Here's how the part is built. I have some questions about the finished solid (model axes, mm). Face numbers are marked on the shaded views. A direction names the side the tool comes from. Give positions to 0.01 mm unless a question says otherwise; leave off trailing zeros. Write each loop counter-clockwise with the first axis right and the second up, starting at its lowest first coordinate (ties: lowest second). Pieces come first, ordered by that corner, then holes. Notation, with made-up numbers: (9.5, -33.75) - (26.5, -33.75) arc R30 cw to (26.5, -10.75) - close; hole circle Ø3 at (-5.75, 29). An arc over 180 degrees is marked (long way). One line per item, written item: value. Start each with the question number.
1) I'm going to push flat-ended pins straight in: P1, Ø2.5, axis at x = 7, z = -3, coming from the +Y side; P2, Ø1.5, axis at y = 1, z = 6.5, coming from the -X side; P3, Ø1, axis at y = 0, z = 5, coming from the -X side. Where does each tip first touch, or does it pass through?
2) Imagine slicing it at B-B on z = 7. Write out the boundary of the cut face in (x, y).
3) Imagine slicing it at A-A on y = -0.8. Count the separate pieces of the cut face and the enclosed holes in it, plus the area to 3 significant figures.
4) On a 3-axis mill with a long thin cutter (end or side, diameter ignored), from which of +Z, -Z, +X, -X, +Y, -Y can I reach the whole of each face in a straight line? I mean the marked faces 1 and 2. Say none if no direction works.
5) Imagine slicing it at D-D on x = 4. Write out the boundary of the cut face in (y, z).
6) Please list where these lines run through material, in increasing order: L1, parallel to X at y = -0.2, z = 0; L2, parallel to X at y = 0.4, z = -3; L3, parallel to X at y = -0.1, z = 7. Write a range as [from, to].
7) Imagine slicing it at C-C on x = 7. Write out the boundary of the cut face in (y, z), plus the area to 3 significant figures.
8) We'd pull the mould along X, two halves only. Please class the marked faces 3, 4 and 5: +X half, -X half, draft (parallel to the pull), parting line (faces both ways), or undercut.
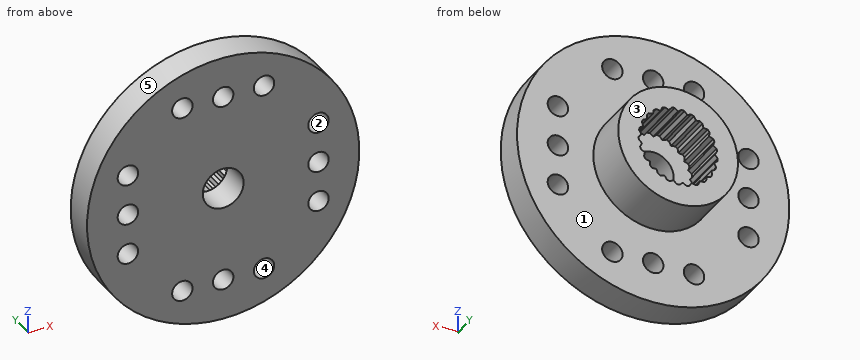
from build123d import *

# Parameters (mm, degrees)
SKETCH2_R           = 6
SKETCH2_R_2         = 1.5
BOSS_EXTRUDE1_DEPTH = 1.15
SKETCH3_R           = 4.4
BOSS_EXTRUDE2_DEPTH = 3.5
SKETCH5_R           = 10
SKETCH5_R_2         = 0.75
SKETCH5_R_3         = 1.5
BOSS_EXTRUDE4_DEPTH = 1.15


with BuildPart() as part:
    # Sketch2 → Boss-Extrude1 (new, symmetric)
    with BuildSketch(Plane(origin=(0, 0, 0), x_dir=(1, 0, 0), z_dir=(0, 1, 0))):
        with Locations(Location((0, 0, 0), (0, 0, 270))):
            Circle(SKETCH2_R)
        with Locations(Location((0, 0, 0), (0, 0, 270))):
            Circle(SKETCH2_R_2, mode=Mode.SUBTRACT)
    extrude(amount=BOSS_EXTRUDE1_DEPTH, both=True)

    # Sketch3 → Boss-Extrude2 (add)
    with BuildSketch(Plane(origin=(0, 1.15, 0), x_dir=(1, 0, 0), z_dir=(0, 1, 0))):
        with Locations(Location((0, 0, 0), (0, 0, 270))):
            Circle(SKETCH3_R)
        with BuildLine():
            Line((0.107421435, 2.898009771), (0.338399731, 2.678709694))
            Line((0.338399731, 2.678709694), (0.61665913, 2.83367809))
            ThreePointArc((0.61665913, 2.83367809), (0.721200673, 2.808891167), (0.824752316, 2.780248841))
            Line((0.824752316, 2.780248841), (0.993936292, 2.510396512))
            Line((0.993936292, 2.510396512), (1.301992734, 2.591295993))
            ThreePointArc((1.301992734, 2.591295993), (1.397085655, 2.541289372), (1.490260976, 2.48779465))
            Line((1.490260976, 2.48779465), (1.587020181, 2.184345885))
            Line((1.587020181, 2.184345885), (1.905517346, 2.186093238))
            ThreePointArc((1.905517346, 2.186093238), (1.985186607, 2.11400902), (2.062131058, 2.039023173))
            Line((2.062131058, 2.039023173), (2.080385755, 1.721044772))
            Line((2.080385755, 1.721044772), (2.389311295, 1.643530205))
            ThreePointArc((2.389311295, 1.643530205), (2.448550984, 1.553897705), (2.504429862, 1.46213237))
            Line((2.504429862, 1.46213237), (2.443033042, 1.149604087))
            Line((2.443033042, 1.149604087), (2.722976028, 0.997698125))
            ThreePointArc((2.722976028, 0.997698125), (2.758063897, 0.896149284), (2.789366126, 0.793370413))
            Line((2.789366126, 0.793370413), (2.652175577, 0.505929549))
            Line((2.652175577, 0.505929549), (2.885546163, 0.289177003))
            ThreePointArc((2.885546163, 0.289177003), (2.894277512, 0.182092507), (2.899036259, 0.074758075))
            Line((2.899036259, 0.074758075), (2.694672167, -0.169534403))
            Line((2.694672167, -0.169534403), (2.866806821, -0.437514174))
            ThreePointArc((2.866806821, -0.437514174), (2.848633027, -0.543405812), (2.826549281, -0.648551587))
            Line((2.826549281, -0.648551587), (2.567852594, -0.834345885))
            Line((2.567852594, -0.834345885), (2.667935462, -1.136714727))
            ThreePointArc((2.667935462, -1.136714727), (2.623998452, -1.234759946), (2.576459817, -1.331110368))
            Line((2.576459817, -1.331110368), (2.279685399, -1.446732346))
            Line((2.279685399, -1.446732346), (2.301427906, -1.764491312))
            ThreePointArc((2.301427906, -1.764491312), (2.234488404, -1.84852957), (2.164481907, -1.930030589))
            Line((2.164481907, -1.930030589), (1.848277186, -1.968215294))
            Line((1.848277186, -1.968215294), (1.790313171, -2.281398419))
            ThreePointArc((1.790313171, -2.281398419), (1.704577232, -2.346149284), (1.616501638, -2.40767989))
            Line((1.616501638, -2.40767989), (1.30073492, -2.366028036))
            Line((1.30073492, -2.366028036), (1.166706475, -2.654956874))
            ThreePointArc((1.166706475, -2.654956874), (1.067561203, -2.696351809), (0.966950626, -2.734045809))
            Line((0.966950626, -2.734045809), (0.671462695, -2.615174535))
            Line((0.671462695, -2.615174535), (0.469791321, -2.861694623))
            ThreePointArc((0.469791321, -2.861694623), (0.363466377, -2.877132634), (0.25664255, -2.888621575))
            Line((0.25664255, -2.888621575), (0, -2.7))
            Line((0, -2.7), (-0.25664255, -2.888621575))
            ThreePointArc((-0.25664255, -2.888621575), (-0.363466377, -2.877132634), (-0.469791321, -2.861694623))
            Line((-0.469791321, -2.861694623), (-0.671462695, -2.615174535))
            Line((-0.671462695, -2.615174535), (-0.966950626, -2.734045809))
            ThreePointArc((-0.966950626, -2.734045809), (-1.067561203, -2.696351809), (-1.166706475, -2.654956874))
            Line((-1.166706475, -2.654956874), (-1.30073492, -2.366028036))
            Line((-1.30073492, -2.366028036), (-1.616501638, -2.40767989))
            ThreePointArc((-1.616501638, -2.40767989), (-1.704577232, -2.346149284), (-1.790313171, -2.281398419))
            Line((-1.790313171, -2.281398419), (-1.848277186, -1.968215294))
            Line((-1.848277186, -1.968215294), (-2.164481907, -1.930030589))
            ThreePointArc((-2.164481907, -1.930030589), (-2.234488404, -1.84852957), (-2.301427906, -1.764491312))
            Line((-2.301427906, -1.764491312), (-2.279685399, -1.446732346))
            Line((-2.279685399, -1.446732346), (-2.576459817, -1.331110368))
            ThreePointArc((-2.576459817, -1.331110368), (-2.623998452, -1.234759946), (-2.667935462, -1.136714727))
            Line((-2.667935462, -1.136714727), (-2.567852594, -0.834345885))
            Line((-2.567852594, -0.834345885), (-2.826549281, -0.648551587))
            ThreePointArc((-2.826549281, -0.648551587), (-2.848633027, -0.543405812), (-2.866806821, -0.437514174))
            Line((-2.866806821, -0.437514174), (-2.694672167, -0.169534403))
            Line((-2.694672167, -0.169534403), (-2.899036259, 0.074758075))
            ThreePointArc((-2.899036259, 0.074758075), (-2.894277512, 0.182092507), (-2.885546163, 0.289177003))
            Line((-2.885546163, 0.289177003), (-2.652175577, 0.505929549))
            Line((-2.652175577, 0.505929549), (-2.789366126, 0.793370413))
            ThreePointArc((-2.789366126, 0.793370413), (-2.758063897, 0.896149284), (-2.722976028, 0.997698125))
            Line((-2.722976028, 0.997698125), (-2.443033042, 1.149604087))
            Line((-2.443033042, 1.149604087), (-2.504429862, 1.46213237))
            ThreePointArc((-2.504429862, 1.46213237), (-2.448550984, 1.553897705), (-2.389311295, 1.643530205))
            Line((-2.389311295, 1.643530205), (-2.080385755, 1.721044772))
            Line((-2.080385755, 1.721044772), (-2.062131058, 2.039023173))
            ThreePointArc((-2.062131058, 2.039023173), (-1.985186607, 2.11400902), (-1.905517346, 2.186093238))
            Line((-1.905517346, 2.186093238), (-1.587020181, 2.184345885))
            Line((-1.587020181, 2.184345885), (-1.490260976, 2.48779465))
            ThreePointArc((-1.490260976, 2.48779465), (-1.397085655, 2.541289372), (-1.301992734, 2.591295993))
            Line((-1.301992734, 2.591295993), (-0.993936292, 2.510396512))
            Line((-0.993936292, 2.510396512), (-0.824752316, 2.780248841))
            ThreePointArc((-0.824752316, 2.780248841), (-0.721200673, 2.808891167), (-0.61665913, 2.83367809))
            Line((-0.61665913, 2.83367809), (-0.338399731, 2.678709694))
            Line((-0.338399731, 2.678709694), (-0.107421435, 2.898009771))
            ThreePointArc((-0.107421435, 2.898009771), (0, 2.9), (0.107421435, 2.898009771))
        make_face(mode=Mode.SUBTRACT)
    extrude(amount=BOSS_EXTRUDE2_DEPTH)

    # Sketch5 → Boss-Extrude4 (add, symmetric)
    with BuildSketch(Plane(origin=(0, 0, 0), x_dir=(1, 0, 0), z_dir=(0, 1, 0))):
        with Locations(Location((0, 0, 0), (0, 0, 270))):
            Circle(SKETCH5_R)
        with Locations(Location((0, 7, 0), (0, 0, 270))):
            Circle(SKETCH5_R_2, mode=Mode.SUBTRACT)
        with Locations(Location((-3, 7, 0), (0, 0, 270))):
            Circle(SKETCH5_R_2, mode=Mode.SUBTRACT)
        with Locations(Location((3, 7, 0), (0, 0, 270))):
            Circle(SKETCH5_R_2, mode=Mode.SUBTRACT)
        with Locations(Location((7, 3, 0), (0, 0, 270))):
            Circle(SKETCH5_R_2, mode=Mode.SUBTRACT)
        with Locations(Location((7, 0, 0), (0, 0, 270))):
            Circle(SKETCH5_R_2, mode=Mode.SUBTRACT)
        with Locations(Location((7, -3, 0), (0, 0, 270))):
            Circle(SKETCH5_R_2, mode=Mode.SUBTRACT)
        with Locations(Location((3, -7, 0), (0, 0, 270))):
            Circle(SKETCH5_R_2, mode=Mode.SUBTRACT)
        with Locations(Location((0, -7, 0), (0, 0, 270))):
            Circle(SKETCH5_R_2, mode=Mode.SUBTRACT)
        with Locations(Location((-3, -7, 0), (0, 0, 270))):
            Circle(SKETCH5_R_2, mode=Mode.SUBTRACT)
        with Locations(Location((-7, -3, 0), (0, 0, 270))):
            Circle(SKETCH5_R_2, mode=Mode.SUBTRACT)
        with Locations(Location((-7, 0, 0), (0, 0, 270))):
            Circle(SKETCH5_R_2, mode=Mode.SUBTRACT)
        with Locations(Location((-7, 3, 0), (0, 0, 270))):
            Circle(SKETCH5_R_2, mode=Mode.SUBTRACT)
        with Locations(Location((0, 0, 0), (0, 0, 270))):
            Circle(SKETCH5_R_3, mode=Mode.SUBTRACT)
    extrude(amount=BOSS_EXTRUDE4_DEPTH, both=True)


solid = part.part
Numbers:
1. P1: y = 1.15
1. P2: x = -8.18
1. P3: x = -8.93
2. outline: (-7.14, -1.15) - (-3.75, -1.15) - (-3.75, 1.15) - (-7.14, 1.15) - close; (-2.25, -1.15) - (-0.75, -1.15) - (-0.75, 1.15) - (-2.25, 1.15) - close; (0.75, -1.15) - (2.25, -1.15) - (2.25, 1.15) - (0.75, 1.15) - close; (3.75, -1.15) - (7.14, -1.15) - (7.14, 1.15) - (3.75, 1.15) - close
3. separate pieces: 1
3. enclosed holes: 13
3. area: 286 mm^2
4. face 1: +Y
4. face 2: +Y, -Y
5. outline: (-1.15, -9.17) - (1.15, -9.17) - (1.15, -1.83) - (4.65, -1.83) - (4.65, 1.83) - (1.15, 1.83) - (1.15, 9.17) - (-1.15, 9.17) - close
6. L1: [-10, -7.75], [-6.25, -1.5], [1.5, 6.25], [7.75, 10]
6. L2: [-9.54, -7.75], [-6.25, 6.25], [7.75, 9.54]
6. L3: [-7.14, -3.75], [-2.25, -0.75], [0.75, 2.25], [3.75, 7.14]
7. outline: (-1.15, -7.14) - (1.15, -7.14) - (1.15, -3.75) - (-1.15, -3.75) - close; (-1.15, -2.25) - (1.15, -2.25) - (1.15, -0.75) - (-1.15, -0.75) - close; (-1.15, 0.75) - (1.15, 0.75) - (1.15, 2.25) - (-1.15, 2.25) - close; (-1.15, 3.75) - (1.15, 3.75) - (1.15, 7.14) - (-1.15, 7.14) - close
7. area: 22.5 mm^2
8. face 3: draft
8. face 4: undercut
8. face 5: parting line
